Check sheet for the drawn part. Datum: minimum x, y, z corner. Units: mm. Give positions to 0.01 mm unless a question says otherwise; leave off trailing zeros. Loops run counter-clockwise (first coordinate to the right, second up) from the corner with the lowest first, then second, coordinate; pieces in that order, holes last. Notation, with made-up numbers: M -2.75,-32 L 9.25,-32 A7 ccw 9.25,-19 Z; hole C -34.5,15.25 d3. An arc over 180 degrees is marked long. Write each question's results on one line, items separated by ' | '. Start each with the question number.
1. Sectioned sample at A-A on x = 2. Record the cut outline in (y, z) (3 decimals).
2. Sectioned sample at B-B on z = 2. Record the cut outline in (x, y) (3 decimals), and give its area (3 significant figures).
3. Sectioned sample at C-C on y = 16. Record the cut outline in (x, z) (3 decimals), and give its area (3 significant figures).
4. Material ranges on line 1 along Z through (x, y) = (2, 0.95) (3 decimals); line 2 along X through (y, z) = (10.5, 2.1), recorded low to high.
5. Draft check along X on the marked faces 1, 2 and 3. Enter one of: pulls with the +X half, pulls with the -X half, needs draft (parallel to the pull), parting line crosses it, or undercut.
6. Go/stop test with flat-tipped pins: pin 1 (2 mm diameter, centred on x = 2, y = 18, fed in from -Z) (3 decimals); pin 2 (1.6 mm diameter, centred on x = 2, z = 2, fed in from -Y); pin 3 (1.5 mm diameter, centred on x = 1, z = 1.5, fed in from -Y). Record where each tip stops, or that it passes through.
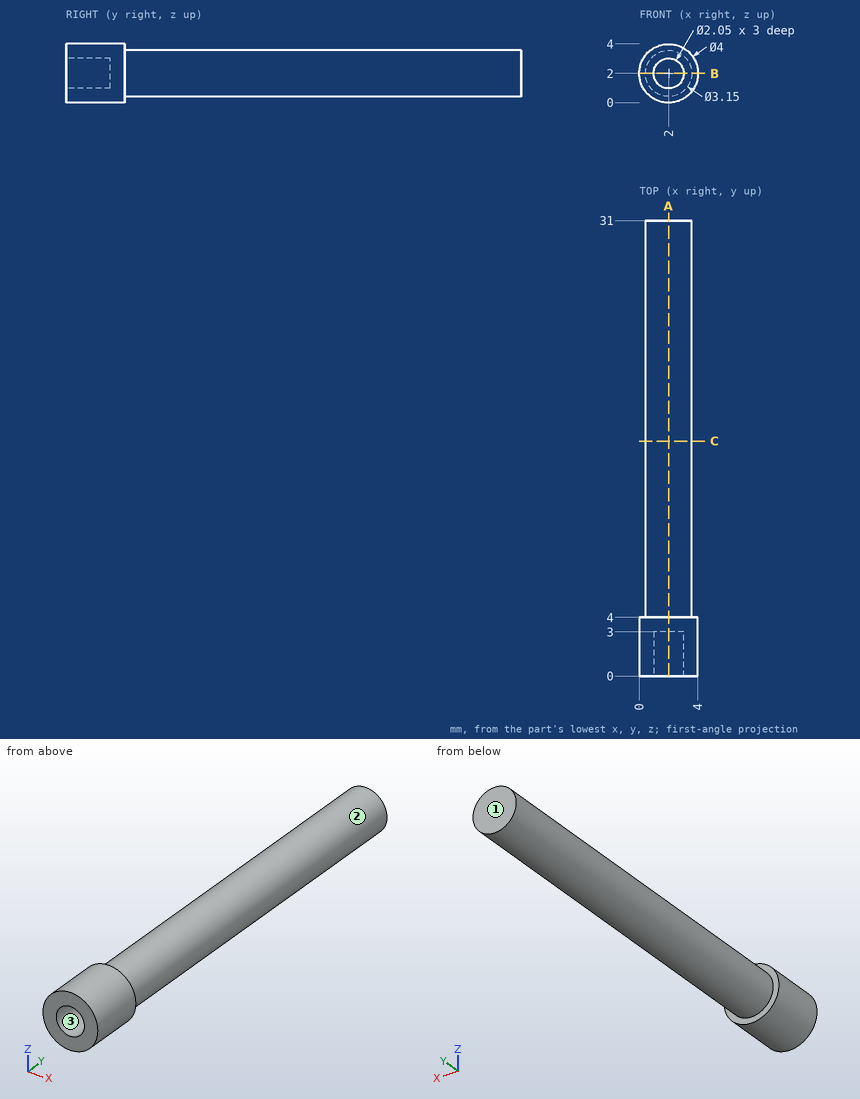
Output values:
1) outline: M 0,0 L 4,0 L 4,0.425 L 31,0.425 L 31,3.575 L 4,3.575 L 4,4 L 0,4 L 0,3.025 L 3,3.025 L 3,0.975 L 0,0.975 Z
2) outline: M 0,0 L 0.975,0 L 0.975,3 L 3.025,3 L 3.025,0 L 4,0 L 4,4 L 3.575,4 L 3.575,31 L 0.425,31 L 0.425,4 L 0,4 Z | area: 94.9 mm2
3) outline: C 2,2 d3.15 | area: 7.79 mm2
4) line 1: 0 to 0.975, 3.025 to 4 | line 2: 0.43 to 3.57
5) face 1: needs draft | face 2: parting line crosses it | face 3: undercut
6) pin 1: z = 0.425 | pin 2: y = 3 | pin 3: y = 0
